Source: CAD feature listing. Evaluate the final solid. Frame: model axes, mm. A direction names the side the tool comes from. Give positions to 0.01 mm unless a question says otherwise; leave off trailing zeros. Write each loop counter-clockwise with the first axis right and the second up, starting at its lowest first coordinate (ties: lowest second). Pieces come first, ordered by that corner, then holes. Notation, with made-up numbers: (26, 31) -> (72, 31) arc R10 ccw to (72, 49) -> close; hole circle Ø6 at (-14, -26.75). An arc over 180 degrees is marked (long way). Write item = value, one per line.
from build123d import *

# Parameters (mm, degrees)
F0_W      = 67.1
F0_H      = 138.3
F1_DEPTH  = 12.7
F2_T      = -2.54
F3_R      = 5.08
F4_W      = 23.2377038337
F4_H      = 8.8934414089
F5_DEPTH  = 12.5
F6_W      = 14.3442638218
F6_H      = 4.4467216358
F7_DEPTH  = 35
F9_DEPTH  = 27.5
F10_W     = 3.4426231869
F10_H     = 14.3442638218
F11_DEPTH = 27.5
F13_DEPTH = 1.5
F15_DEPTH = 27.5


with BuildPart() as f1:
    # F0 (on Front) → F1 (new body, symmetric)
    with BuildSketch(Plane.XZ):
        Rectangle(F0_W, F0_H)
    extrude(amount=F1_DEPTH, both=True)

    # F2
    f2_openings = [f1.faces().sort_by_distance(p)[0] for p in [
        (0, -12.7, 0),
    ]]
    offset(amount=F2_T, openings=f2_openings)

    # F3
    f3_edges = [f1.edges().sort_by_distance(p)[0] for p in [
        (33.55, 0, 69.15),
        (33.55, 0, -69.15),
        (-33.55, 0, 69.15),
        (-33.55, 0, -69.15),
    ]]
    fillet(f3_edges, radius=F3_R)

    # F4 (on face) → F5 (cut, symmetric)
    with BuildSketch(Plane.XZ.offset(-10.16)):
        with Locations((15.061476035, 59.0983647853)):
            Rectangle(F4_W, F4_H)
    extrude(amount=F5_DEPTH, both=True, mode=Mode.SUBTRACT)

    # F6 (on face) → F7 (cut, symmetric)
    with BuildSketch(Plane(origin=(0, 0, -69.15), x_dir=(1, 0, 0), z_dir=(0, 0, -1))):
        with Locations((-0.5737706088, 2.2233608179)):
            Rectangle(F6_W, F6_H)
    extrude(amount=F7_DEPTH, both=True, mode=Mode.SUBTRACT)

    # F8 (on face) → F9 (cut, symmetric)
    with BuildSketch(Plane(origin=(-33.55, 0, 0), x_dir=(0, -1, 0), z_dir=(-1, 0, 0))):
        with BuildLine():
            add(Edge.make_bspline(
                [(0, 60.676228255), (-7.550774062, 60.676228255), (-3.775387031, 39.1598381102), (0, 17.6434479654), (3.775387031, 39.1598381102), (7.550774062, 60.676228255), (0, 60.676228255)],
                knots=[0, 0, 0, 2.0943951024, 2.0943951024, 4.1887902048, 4.1887902048, 6.2831853072, 6.2831853072, 6.2831853072], degree=2, weights=[1, 0.5, 1, 0.5, 1, 0.5, 1]))
        make_face()
    extrude(amount=F9_DEPTH, both=True, mode=Mode.SUBTRACT)

    # F10 (on face) → F11 (cut, symmetric)
    with BuildSketch(Plane.YZ.offset(33.55)):
        with Locations((-1.7213115934, 46.9057392329)):
            Rectangle(F10_W, F10_H)
    extrude(amount=F11_DEPTH, both=True, mode=Mode.SUBTRACT)

    # F12 (on face) → F13 (cut, symmetric)
    with BuildSketch(Plane(origin=(0, 12.7, 0), x_dir=(-1, 0, 0), z_dir=(0, 1, 0))):
        Polygon((-5.2382490833, 6.1278682367), (-9.4672134146, 6.7418036051), (-15.491804108, -23.0942647904), (4.0163947269, -23.0942647904), (4.0163947269, -19.0778691322), (-10.3278690949, -19.0778691322), align=None)
    extrude(amount=F13_DEPTH, both=True, mode=Mode.SUBTRACT)

    # F14 (on face) → F15 (cut, symmetric)
    with BuildSketch(Plane(origin=(0, 12.7, 0), x_dir=(-1, 0, 0), z_dir=(0, 1, 0))):
        Polygon((-12.711224328, 6.7418036051), (-18.3606576174, 6.7418036051), (-11.2235988457, -1.9564862073), (-10.1078801099, 3.5689780455), align=None)
        Polygon((-6.6146179771, -0.6884349019), (-7.730336713, -6.2138991547), (0, -15.635246411), (16.0655751824, 6.7418036051), (10.901639238, 6.7418036051), (0, -8.7500000373), align=None)
    extrude(amount=F15_DEPTH, both=True, mode=Mode.SUBTRACT)


solid = f1.part
1) Cut plane A-A (y = 6). Return the cut outline in (x, z), then the cut area to 3 significant figures.
Computed:
outline = (-33.55, -64.07) arc R5.08 ccw to (-28.47, -69.15) -> (28.47, -69.15) arc R5.08 ccw to (33.55, -64.07) -> (33.55, 64.07) arc R5.08 ccw to (28.47, 69.15) -> (-28.47, 69.15) arc R5.08 ccw to (-33.55, 64.07) -> close; hole (-31.01, -66.61) -> (31.01, -66.61) -> (31.01, 66.61) -> (-31.01, 66.61) -> close
area = 995 mm²
2) Cut plane C-C (x = -24). Return the cut outline in (y, z), then the cut area to 3 significant figures.
Computed:
outline = (-12.7, -69.15) -> (12.7, -69.15) -> (12.7, 69.15) -> (-12.7, 69.15) -> (-12.7, 66.61) -> (10.16, 66.61) -> (10.16, -66.61) -> (-12.7, -66.61) -> close
area = 467 mm²
3) Contact query for flat-ended pins moving along their axis: pin 1 (0.8 mm diameter, centred on y = -2, z = -67.5, fed in from +X); pin 2 (18.5 mm diameter, centred on x = -4.5, z = 12.5, fed in from -Y). Output: stop coordinate, or through.
Computed:
pin_1 = 32.55
pin_2 = 10.16
4) Material intervals for L1, parallel to X at y = 6, z = 52.5; L2, parallel to Z at x = 8, y = -3.5, sorted ascending.
Computed:
L1 = -33.55 to -31.01, 31.01 to 33.55
L2 = -69.15 to -66.61, 66.61 to 69.15
5) Draft query along Z for faces 1 (the cylindrical face through (32.101, -0.178, -67.622)), 2 (the flat face through (-7.746, -2, -68)), 3 (the flat face through (32, -3.443, 47)), 4 (the flat face through (13.33, 11.96, -12.38)). Return one class per face: pulls with the +Z half, pulls with the -Z half, needs draft (parallel to the pull), parting line crosses it, or undercut.
Computed:
face_1 = pulls with the -Z half
face_2 = needs draft
face_3 = undercut
face_4 = undercut
6) Access query for faces 5 (the flat face through (6.598, -2, -68)), 6 (the flat face through (0, -1, 66.61)), 7 (the flat face through (32, -2, 39.734)), 8 (the flat face through (11.39, 11.41, 5.13)). Directions: +Z, -Z, +X, -X, +Y, -Y. A direction counts if a zero-diameter tool reaches every point of the face in a straight line with its end or side. Return the directions, or none.
Computed:
face_5 = -Z
face_6 = -Y
face_7 = +X, -X
face_8 = +Y, -Y
7) Cut plane D-D (z = 9.5). Return the cut outline in (x, y), then the cut area to 3 significant figures.
Computed:
outline = (-33.55, -12.7) -> (-31.01, -12.7) -> (-31.01, 10.16) -> (31.01, 10.16) -> (31.01, -12.7) -> (33.55, -12.7) -> (33.55, 12.7) -> (-33.55, 12.7) -> close
area = 287 mm²
8) Cut plane B-B (x = -2). Return the cut outline in (y, z).
Computed:
outline = (-12.7, -69.15) -> (-4.45, -69.15) -> (-4.45, -66.61) -> (-12.7, -66.61) -> close; (-12.7, 66.61) -> (10.16, 66.61) -> (10.16, -5.91) -> (12.7, -5.91) -> (12.7, 69.15) -> (-12.7, 69.15) -> close; (0, -69.15) -> (12.7, -69.15) -> (12.7, -23.09) -> (11.2, -23.09) -> (11.2, -19.08) -> (12.7, -19.08) -> (12.7, -12.85) -> (10.16, -12.85) -> (10.16, -66.61) -> (0, -66.61) -> close
